Part model, mm, in its own coordinate system. A direction names the side the tool comes from. Round coordinates to 2 decimals unless told otherwise and drop trailing zeros. Loops run counter-clockwise (first coordinate to the right, second up) from the corner with the lowest first, then second, coordinate; pieces in that order, holes last. Notation, with made-up numbers: M -24,36 L -17,36 A27 ccw -17,70 Z; hole C 14.5,48 d11. An arc over 180 degrees is marked long. Write each question's results on one line, items separated by ' | '.
Solid Edge part; units mm, degrees
sketch "Sketch1" plane through (0, 0, 0) normal (0, -1, 0) x (1, 0, 0)
  line L0 (3.1, 8) -> (3.6, 8)
  line L1 (3.6, 8) -> (3.6, 6.2)
  line L2 (4.8, 6.8) -> (3.6, 6.2)
  line L3 (4.8, 7.2) -> (4.8, 6.8)
  line L4 (4.8, 7.2) -> (5.6, 7.2)
  line L5 (5.6, 7.2) -> (5.6, 5.2)
  line L6 (4, 4.4) -> (5.6, 5.2)
  line L7 (4, 4.4) -> (4, 3.6)
  line L8 (4, 3.6) -> (5.6, 2.8)
  line L9 (5.6, 0.8) -> (5.6, 2.8)
  line L10 (5.6, 0.8) -> (4.8, 0.8)
  line L11 (4.8, 0.8) -> (4.8, 1.2)
  line L12 (3.6, 1.8) -> (4.8, 1.2)
  line L13 (3.6, 0) -> (3.6, 1.8)
  line L14 (3.6, 0) -> (3.1, 0)
  line L15 (3.1, 0.8) -> (3.1, 0)
  line L16 (2.4, 0.8) -> (3.1, 0.8)
  line L17 (2.4, 7.2) -> (2.4, 0.8)
  line L18 (2.4, 7.2) -> (3.1, 7.2)
  line L19 (3.1, 8) -> (3.1, 7.2)
revolve "RevolvedProtrusion1" add sketch "Sketch1" angle 360 about axis through (0, 0, 54) along (0, 0, -1)
sketch "Sketch2" plane through (0, 0, 7.2) normal (0, 0, 1) x (1, 0, 0)
  line L0 (4.8, 0) -> (4.8, 0.6)
  line L1 (4.8, 0.6) -> (3.5496, 0.6)
  line L2 (3.5496, 0.6) -> (3.5496, -0.6)
  line L3 (3.5496, -0.6) -> (4.8, -0.6)
  line L4 (4.8, -0.6) -> (4.8, 0)
  line L5 (-3.5496, 0.6) -> (-3.5496, -0.6)
  line L6 (-4.8, -0.6) -> (-3.5496, -0.6)
  line L7 (-4.8, 0) -> (-4.8, -0.6)
  line L8 (-4.8, 0.6) -> (-4.8, 0)
  line L9 (-3.5496, 0.6) -> (-4.8, 0.6)
  line L10 (0, 4.8) -> (-0.6, 4.8)
  line L11 (-0.6, 4.8) -> (-0.6, 3.5496)
  line L12 (-0.6, 3.5496) -> (0.6, 3.5496)
  line L13 (0.6, 3.5496) -> (0.6, 4.8)
  line L14 (0.6, 4.8) -> (0, 4.8)
  line L15 (0, -4.8) -> (-0.6, -4.8)
  line L16 (-0.6, -4.8) -> (-0.6, -3.5496)
  line L17 (-0.6, -3.5496) -> (0.6, -3.5496)
  line L18 (0.6, -3.5496) -> (0.6, -4.8)
  line L19 (0.6, -4.8) -> (0, -4.8)
extrude "Protrusion1" add sketch "Sketch2" against normal blind 1
mirror "Mirror1" about plane through (0, 0, 4) normal (0, 0, 1) of "Protrusion1"
Item 1: Which spindle directions (+Z, -Z, +X, -X, +Y, -Y) get a long thin tool onto all of the face, cutting with end or side? Do faces 1 (the flat face through (4, 0.6, 7)), 2 (the flat face through (-0.6, -4, 1)). Say none if no direction does.
Filled sheet:
face 1: +Z | face 2: -Z
Item 2: Band-saw the part on D-D on z = 4. Give the cut face in (x, y).
Filled sheet:
outline: C 0,0 d8; hole C 0,0 d4.8
Item 3: Two-plate mould, pull along Y, no slides. Class faces 3 (the cylindrical face through (1.661, -3.194, 0.913)), 4 (the flat face through (-4, 0, 0.8)): +Y half, -Y half, draft (parallel to the pull), parting line (faces both ways), or undercut.
Filled sheet:
face 3: undercut | face 4: draft
Item 4: Band-saw the part on C-C on z = 6.5. Give the cut face in (x, y), and give its area (3 significant figures).
Filled sheet:
outline: C 0,0 d11.2; hole M -4.16,-0.6 A4.2 ccw -0.6,-4.16 L -0.6,-3.55 A3.6 cw -3.55,-0.6 Z; hole M -4.16,0.6 L -3.55,0.6 A3.6 cw -0.6,3.55 L -0.6,4.16 A4.2 ccw Z; hole C 0,0 d4.8; hole M 0.6,-4.16 A4.2 ccw 4.16,-0.6 L 3.55,-0.6 A3.6 cw 0.6,-3.55 Z; hole M 0.6,3.55 A3.6 cw 3.55,0.6 L 4.16,0.6 A4.2 ccw 0.6,4.16 Z | area: 68.6 mm^2
Item 5: Wall check: L1, parallel to Y at x = 0, z = 3.75; L2, parallel to Y at x = 0, z = 0.6. Give the ranges that are in metal, low to high.
Filled sheet:
L1: -4 to -2.4, 2.4 to 4 | L2: -3.6 to -3.1, 3.1 to 3.6
Item 6: Drop flat-ended pins along their axis: P1, Ø3, axis at y = 3.5, z = 5.5, coming from the -X side; P2, Ø1.9, axis at x = 1, y = 1.5, coming from the -Z side; P3, Ø0.5, axis at x = -4.5, z = 1.5, coming from the +Y side. Give the stop position or say it passes through.
Filled sheet:
P1: x = -5.23 | P2: z = 0.8 | P3: y = 3.65
